The model under review builds one solid part; all positions refer to its coordinate system, in mm. Give positions to 0.01 mm unless a question says otherwise; leave off trailing zeros.
Autodesk Inventor part; units mm, degrees
ref_plane "YZ Plane" through (0, 0, 0) normal (1, 0, 0) x (0, 1, 0)
ref_plane "XZ Plane" through (0, 0, 0) normal (0, 1, 0) x (-1, 0, 0)
ref_plane "XY Plane" through (0, 0, 0) normal (0, 0, 1) x (1, 0, 0)
sketch "Sketch1" plane through (0, 0, 0) normal (1, 0, 0) x (0, 1, 0)
  line L0 (0, 4.8581) -> (0, -4.8581)
  line L1 (0, 4.8581) -> (1000, -196.5631)
  line L2 (1000, -196.5631) -> (1000, -206.2794)
  line L3 (1000, -206.2794) -> (0, -4.8581)
  line L4 (0, 4.8581) -> (-1.8808, -4.4793) construction
  line L5 (-1.8808, -4.4793) -> (0, -4.8581) construction
  point P0 (0, 0)
  point P1 (0, 0)
  dimension "d0" = 9.525
  dimension "d1" = 1000
  dimension "d9" = 211.1375
  dimension "d10" = 78.612
extrude "Extrusion1" add sketch "Sketch1" along normal mid plane 38.1
sketch "Sketch2" plane through (0, 0, 0) normal (0, 0, 1) x (1, 0, 0)
  circle A0 centre (0, 980.95) radius 6.35
  circle A1 centre (0, 980.95) radius 19.05
  line L0 (19.05, 1000) -> (19.05, 0)
  line L1 (-19.05, 1000) -> (19.05, 1000)
  line L2 (-19.05, 1000) -> (-19.05, 980.95)
  point P0 (0, 0)
  point P1 (0, 1000)
  point P2 (19.05, 980.95)
  dimension "d5" = 38.1
  dimension "d6" = 12.7
extrude "Extrusion2" cut sketch "Sketch2" along normal through all both and the other way through all contours A0 | L2 L1 A1 | A1 L1 L0
sketch "Sketch3" plane through (-19.05, 0, 4.8581) normal (0, 0.1974556, 0.9803118) x (1, 0, 0)
  line L0 (0, 1002.5695) -> (0, 1.9185)
  line L1 (0, 493.095) -> (9.525, 495)
  line L2 (9.525, 495) -> (9.525, 465)
  line L3 (9.525, 465) -> (0, 466.905)
  line L4 (38.1, 0) -> (0, 0)
  line L5 (0, 493.095) -> (9.525, 493.095) construction
  point P0 (19.05, 0.9593)
  point P1 (9.525, 480)
  dimension "d11" = 9.525
  dimension "d12" = 480
  dimension "d14" = 1.905
  dimension "d15" = 30
extrude "Extrusion3" cut sketch "Sketch3" against normal blind 10
mirror "Mirror1" about plane through (0, 0, 0) normal (1, 0, 0) of "Extrusion3"
sketch "Sketch4" plane through (-19.05, 0, 4.8581) normal (0, 0.1974556, 0.9803118) x (1, 0, 0)
  circle A0 centre (19.05, 51.7593) radius 12.7
  line L0 (38.1, 466.905) -> (38.1, 0)
  circle A1 centre (19.05, 89.8593) radius 12.7
  circle A2 centre (19.05, 127.9593) radius 12.7
  circle A3 centre (19.05, 166.0593) radius 12.7
  circle A4 centre (19.05, 204.1593) radius 12.7
  circle A5 centre (19.05, 242.2593) radius 12.7
  circle A6 centre (19.05, 280.3593) radius 12.7
  circle A7 centre (19.05, 318.4593) radius 12.7
  circle A8 centre (19.05, 356.5593) radius 12.7
  circle A9 centre (19.05, 394.6593) radius 12.7
  circle A10 centre (19.05, 432.7593) radius 12.7
  point P0 (19.05, 0.9593)
  dimension "d18" = 25.4
  dimension "d19" = 50.8
  dimension "d22" = 38.1
extrude "Extrusion4" cut sketch "Sketch4" against normal through all
ref_plane "Work Plane1" through (-9.525, 470.5497, -89.9205) normal (0, 0.9803118, -0.1974556) x (-1, 0, 0)
mirror "Mirror2" about plane through (-9.525, 470.5497, -89.9205) normal (0, 0.9803118, -0.1974556) of "Extrusion4"
equation "\"d14\" = 0.2 * d11"
properties part number "UPRIGHTS_TREBUCHET" material "Wood (Birch)"
1. Draft analysis for pull direction X (two halves, no side actions). For faces 1 (the cylindrical face through (12.114, 893.172, -179.836)), 2 (the flat face through (-19.05, 228, -46)), 3 (the flat face through (19.05, 228, -46)), 4 (the cylindrical face through (11.73, 585.86, -117.94)), state which applies: pulls with the +X half, pulls with the -X half, needs draft (parallel to the pull), parting line crosses it, or undercut.
2. Take a section at A-A (x = 0). Count the separate pieces of the cut face and the enclosed holes in it, and give its area (3 significant figures).
3. Insertion check: pin 1 (6 mm diameter, centred on y = 280, z = -65.5, fed in from +X); pin 2 (1 mm diameter, centred on x = -10, y = 870, fed in from -Z); pin 3 (5 mm diameter, centred on x = -6.5, y = 437, fed in from -Z); pin 4 (12 mm diameter, centred on y = 469.5, z = -94, fed in from -X) (3 decimals). Each pin has a flat end and moves straight along its axis. Give the tip position at first contact, or say it passes through.
4. To check wall thickness, follow line 1 (X direction, y = 980, z = -198); line 2 (Z direction, x = 12, y = 673); line 3 (Z direction, x = -14.5, y = 257.5). State the ranges of each line that lie inside material, in increasing order.
Answer:
1. face 1: undercut
1. face 2: pulls with the -X half
1. face 3: pulls with the +X half
1. face 4: undercut
2. separate pieces: 24
2. enclosed holes: 0
2. area: 4,270 mm2
3. pin 1: passes through
3. pin 2: stops at z = -180.2
3. pin 3: stops at z = -93.38
3. pin 4: stops at x = -9.525
4. line 1: x = -19.05 to -6.28, 6.28 to 19.05
4. line 2: z = -140.41 to -130.7
4. line 3: z = -56.72 to -47.01
